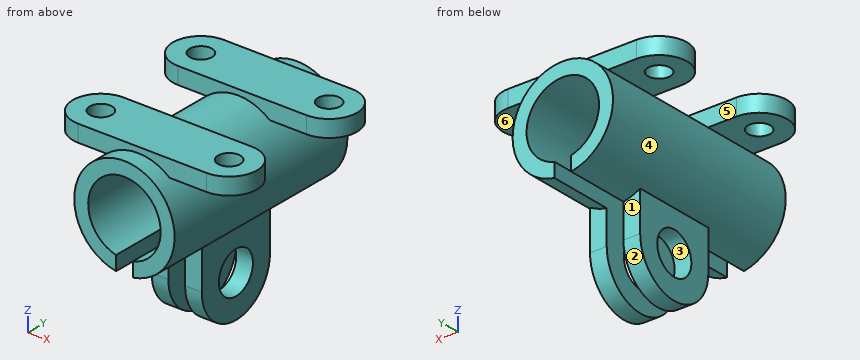
Autodesk Inventor part; units mm, degrees
ref_plane "Work Plane1" through (3.7455, 17.7471, -79.3706) normal (1, 0, 0) x (0, 1, 0)
ref_plane "Work Plane2" through (-3.7545, -157.2529, -79.3706) normal (1, 0, 0) x (0, 0, -1)
ref_plane "YZ Plane" through (0, 0, 0) normal (1, 0, 0) x (0, 1, 0)
sketch "Sketch1" plane through (0, 0, 0) normal (0, 0, 1) x (1, 0, 0)
  line L0 (-57.5, -7.2529) -> (57.5, -7.2529) construction
  line L1 (-57.5, -32.2529) -> (57.5, -32.2529)
  line L2 (57.5, 17.7471) -> (-57.5, 17.7471)
  arc A0 (-57.5, 17.7471) -> (-57.5, -32.2529) centre (-57.5, -7.2529) ccw
  arc A1 (57.5, -32.2529) -> (57.5, 17.7471) centre (57.5, -7.2529) ccw
  circle A2 centre (-57.5, -7.2529) radius 10
  circle A3 centre (57.5, -7.2529) radius 10
  line L3 (-57.5, -117.2529) -> (57.5, -117.2529) construction
  line L4 (-57.5, -142.2529) -> (57.5, -142.2529)
  line L5 (57.5, -92.2529) -> (-57.5, -92.2529)
  arc A4 (-57.5, -92.2529) -> (-57.5, -142.2529) centre (-57.5, -117.2529) ccw
  arc A5 (57.5, -142.2529) -> (57.5, -92.2529) centre (57.5, -117.2529) ccw
  circle A6 centre (-57.5, -117.2529) radius 10
  circle A7 centre (57.5, -117.2529) radius 10
  point P0 (0, 0)
  point P1 (0, -7.2529)
  point P2 (0, -117.2529)
  point P3 (82.5, -117.2529)
  point P4 (-82.5, -117.2529)
  dimension "d0" = 115
  dimension "d1" = 25
  dimension "d2" = 20
  dimension "d3" = 20
  dimension "d4" = 115
  dimension "d5" = 25
  dimension "d6" = 20
  dimension "d7" = 20
  dimension "d8" = 110
  dimension "d11" = 165
extrude "Extrusion1" add sketch "Sketch1" along normal blind 15
sketch "Sketch2" plane through (0, 0, 0) normal (0, 0, -1) x (-1, 0, 0)
  point P0 (0, 0)
sketch "Sketch3" plane through (0, 0, 0) normal (0, 0, -1) x (-1, 0, 0)
  point P0 (0, 0)
sketch "Sketch4" plane through (-57.5, 17.7471, 0) normal (0, 1, 0) x (1, 0, 0)
  arc A0 (46.2455, 79.3706) -> (61.2455, 79.3706) centre (53.7455, 35) ccw
  line L0 (115, 0) -> (0, 0)
  arc A1 (46.2455, 66.6228) -> (61.2455, 66.6228) centre (53.7455, 35) ccw
  line L1 (46.2455, -10) -> (61.2455, 80) construction
  line L2 (61.2455, -10) -> (46.2455, 80) construction
  line L3 (46.2455, 79.3706) -> (46.2455, 66.6228)
  line L4 (61.2455, 66.6228) -> (61.2455, 79.3706)
  point P0 (57.5, 0)
  dimension "d12" = 90
  dimension "d13" = 35
  dimension "d14" = 65
  dimension "d15" = 15
  dimension "d16" = 90
extrude "Extrusion2" add sketch "Sketch4" along normal blind 15 and the other way blind 175
sketch "Sketch5" plane through (0, 0, 0) normal (1, 0, 0) x (0, 1, 0)
  point P0 (0, 0)
ref_plane "Work Plane1" through (3.7455, 17.7471, -79.3706) normal (1, 0, 0) x (0, 1, 0)
sketch "Sketch6" plane through (3.7455, 17.7471, -79.3706) normal (1, 0, 0) x (0, 1, 0)
  circle A0 centre (-80, -30.1908) radius 18.75
  arc A1 (-117.5, -30.1908) -> (-42.5, -30.1908) centre (-80, -30.1908) ccw
  line L0 (-117.5, -30.1908) -> (-117.5, 12.3826)
  line L1 (-117.5, 12.3826) -> (-42.5, 12.3826)
  line L2 (-42.5, 12.3826) -> (-42.5, -30.1908)
  point P0 (-17.7471, 79.3706)
  dimension "d21" = 37.5
  dimension "d22" = 75
extrude "Extrusion3" add sketch "Sketch6" along normal blind 15
ref_plane "Work Plane2" through (-3.7545, -157.2529, -79.3706) normal (1, 0, 0) x (0, 0, -1)
mirror "Mirror1" about plane through (-3.7545, -157.2529, -79.3706) normal (1, 0, 0) of "Extrusion3"
properties part number "cad@68"
Could you check a few things on this model? Use its own coordinates, in mm. Face numbers are marked on the shaded views. A direction names the side the tool comes from. Give positions to 0.01 mm unless a question says otherwise; leave off trailing zeros. Loops run counter-clockwise (first coordinate to the right, second up) from the corner with the lowest first, then second, coordinate; pieces in that order, holes last. Notation, with made-up numbers: M 89.25,77.5 L 115.25,77.5 A14 ccw 115.25,97.5 Z; hole C 76.5,12.25 d10. An arc over 180 degrees is marked long. Answer as a JSON object with one key per item and string values.
Q1. For the marked faces 4, 5 and 6, which set-ups out of +Z, -Z, +X, -X, +Y, -Y let a thin tool reach every point of the face, with its end or its side?
Values found:
{"face 4": "none", "face 5": "+Z", "face 6": "+X, +Y, -Y"}
Q2. If we mould it in two halves opening along Z, with no side actions, what happens to the marked faces 1, 2 and 3? For each: pulls with the +Z half, pulls with the -Z half, needs draft (parallel to the pull), parting line crosses it, or undercut.
Values found:
{"face 1": "needs draft", "face 2": "pulls with the -Z half", "face 3": "undercut"}
Q3. If I drill on probe 1 along Y at (x, z) = (-57.5, 5); probe 2 along X at (y, z) = (-77.5, -131); probe 3 along X at (y, z) = (-26, -35), over which ranges is the centre line in solid material (lowest first)? Write a range as [from, to].
Values found:
{"probe 1": "y = [-142.25, -127.25], [-107.25, -92.25], [-32.25, -17.25], [2.75, 17.75]", "probe 2": "x = [-26.25, -11.25], [3.75, 18.75]", "probe 3": "x = [-48.75, -36.25], [28.75, 41.25]"}
Q4. Suppose I cut it at C-C, the plane x = 13. List the corners of the cut face in (y, z) for me.
Values found:
{"outline": "M -157.25,-76.76 L -99.75,-76.76 L -99.75,-109.56 A37.5 ccw -24.75,-109.56 L -24.75,-76.76 L 32.75,-76.76 L 32.75,-62.85 L -157.25,-62.85 Z; M -157.25,-7.15 L 32.75,-7.15 L 32.75,6.76 L 17.75,6.76 L 17.75,15 L -32.25,15 L -32.25,6.76 L -92.25,6.76 L -92.25,15 L -142.25,15 L -142.25,6.76 L -157.25,6.76 Z; hole C -62.25,-109.56 d37.5"}
Q5. Suppose I cut it at B-B, the plane y = -49.5. List the corners of the cut face in (x, z) for me, plus the area to 3 significant figures.
Values found:
{"outline": "M -26.25,-144.83 L -11.25,-144.83 L -11.25,-123.31 L -26.25,-123.31 Z; M -26.25,-95.82 L -11.25,-95.82 L -11.25,-66.62 A32.5 cw long 3.75,-66.62 L 3.75,-95.82 L 18.75,-95.82 L 18.75,-73.97 A45 ccw long -26.25,-73.97 Z; M 3.75,-144.83 L 18.75,-144.83 L 18.75,-123.31 L 3.75,-123.31 Z", "area": "4,060 mm²"}
Q6. Suppose I cut it at D-D, the plane x = 50.5. List the corners of the cut face in (y, z) for me, plus the area to 3 significant figures.
Values found:
{"outline": "M -142.25,0 L -124.39,0 L -124.39,15 L -142.25,15 Z; M -110.11,0 L -92.25,0 L -92.25,15 L -110.11,15 Z; M -32.25,0 L -14.39,0 L -14.39,15 L -32.25,15 Z; M -0.11,0 L 17.75,0 L 17.75,15 L -0.11,15 Z", "area": "1,070 mm²"}
Q7. Suppose I cut it at A-A, the plane z = -82. List the corners of the cut face in (x, y) for me.
Values found:
{"outline": "M -26.25,-99.75 L -11.25,-99.75 L -11.25,-24.75 L -26.25,-24.75 Z; M 3.75,-99.75 L 18.75,-99.75 L 18.75,-24.75 L 3.75,-24.75 Z"}
Q8. For P1, Ø5, axis at y = -52, z = -85.5, coming from the +X side; P2, Ø5, axis at x = -8.5, y = -118.5, coming from the -Z side; P3, Ø8, axis at x = 53.5, y = -119.5, coming from the -Z side; P4, Ø15, axis at x = -52.5, y = -127.5, coming from the -Z side, each with a flat end and sliding along its axis, tell me the tip position at first contact or that it passes through.
Values found:
{"P1": "stops at x = 18.75", "P2": "stops at z = -3.32", "P3": "passes through", "P4": "stops at z = -52.99"}
